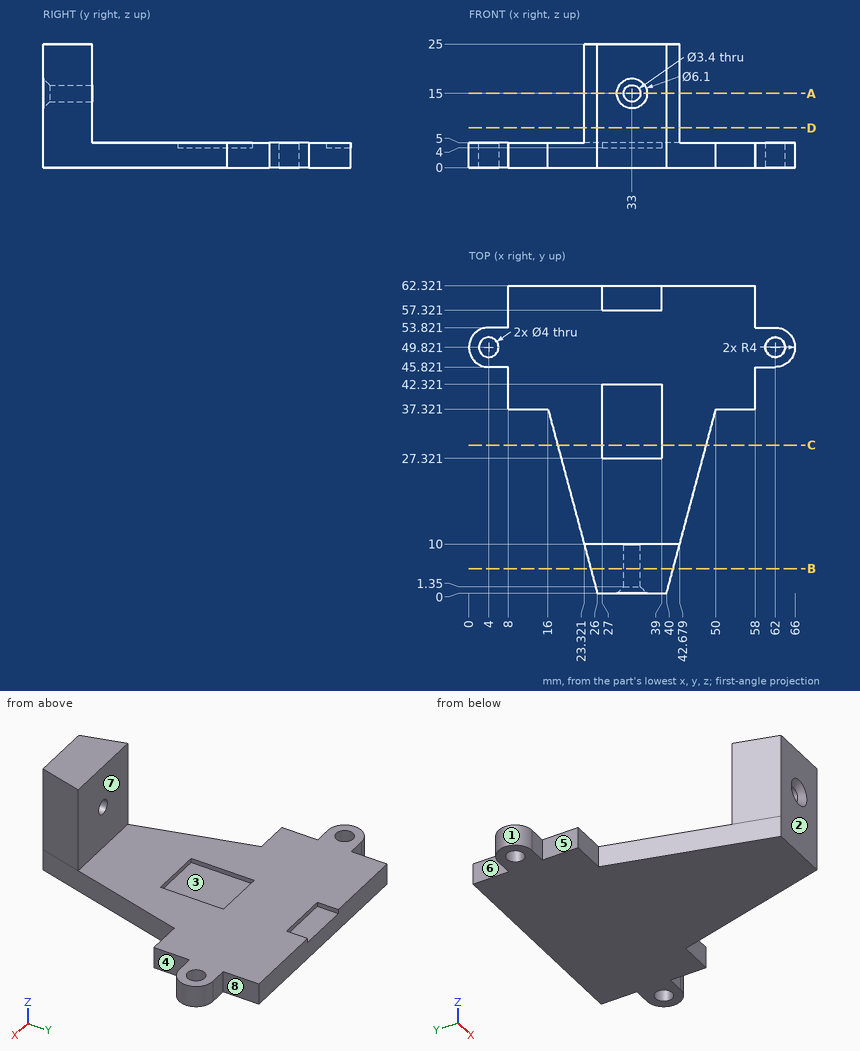
Answer from the drawing. Dimensions are ordinates in mm from the lowest x, y and z of the part. A direction names the side the tool comes from. Give positions to 0.01 mm unless a question says otherwise; leave off trailing zeros. Order: outer loops, then holes, each group sorted by start corner. A loop starts at its lowest first (then second) coordinate and runs counter-clockwise, first axis right, second up. Notation, with made-up numbers: (18.5, -17.5) - (38.5, -17.5) arc R25 ccw to (38.5, 11.5) - close; hole circle Ø11 at (20.25, 45.25). An arc over 180 degrees is marked (long way). One line per item, written item: value. Start each with the question number.
1. Which of the six approach directions +Z, -Z, +X, -X, +Y, -Y give full straight-line access (tool end or side, diameter ignored) to the marked faces 4, 5, 6, 7 and 8?
2. Section D-D, the plane z = 8 is taken. Write down the section's boundary in (x, y), then the cut area to 3 significant figures.
3. For a pull along X with two mould halves and no side action, classify the marked faces 1, 2 and 3 as released by +X, released by -X, zero draft, split by the parting line, or undercut.
4. Consider line 1 (Y direction, x = 62, z = 3.15); line 2 (Z direction, x = 33, y = 7); line 3 (Z direction, x = 46, y = 31). Determine where each line is inside the solid, lowest interval first.
5. Each of these flat-tipped pins is pushed along its axis until it touches: pin 1 Ø5.5 at (x, z) = (11, 3.5) entering from -Y; pin 2 Ø2.5 at (y, z) = (43, 2) entering from -X; pin 3 Ø2.5 at (y, z) = (60, 3.5) entering from +X. Where does it stop, or does it pass through?
6. Section B-B, the plane y = 5 is taken. Write down the section's boundary in (x, z).
7. Section C-C, the plane y = 30 is taken. Write down the section's boundary in (x, z).
8. Section A-A, the plane z = 15 is taken. Write down the section's boundary in (x, y).
Filled sheet:
1. face 4: +Z, -Z, +X, -Y
1. face 5: +Z, -Z, -X, -Y
1. face 6: +Z, -Z, -X, +Y
1. face 7: +Z, +X, -X, +Y
1. face 8: +Z, -Z, +X, +Y
2. outline: (23.32, 10) - (26, 0) - (40, 0) - (42.68, 10) - close
2. area: 167 mm²
3. face 1: released by -X
3. face 2: zero draft
3. face 3: undercut
4. line 1: 45.82 to 47.82, 51.82 to 53.82
4. line 2: 0 to 13.3, 16.7 to 25
4. line 3: 0 to 5
5. pin 1: y = 37.32
5. pin 2: x = 8
5. pin 3: x = 58
6. outline: (24.66, 0) - (41.34, 0) - (41.34, 25) - (24.66, 25) - close; hole circle Ø3.4 at (33, 15)
7. outline: (17.96, 0) - (48.04, 0) - (48.04, 5) - (39, 5) - (39, 4) - (27, 4) - (27, 5) - (17.96, 5) - close
8. outline: (23.32, 10) - (26, 0) - (29.95, 0) - (31.3, 1.35) - (31.3, 10) - close; (34.7, 1.35) - (36.05, 0) - (40, 0) - (42.68, 10) - (34.7, 10) - close
